Verification items for this drawing (mm, ordinates from the low corner). A direction names the side the tool comes from. Round coordinates to 2 decimals unless told otherwise and drop trailing zeros. Loops run counter-clockwise (first coordinate to the right, second up) from the corner with the lowest first, then second, coordinate; pieces in that order, holes last. Notation, with made-up numbers: M -10.5,30.25 L 45.5,30.25 A19 ccw 45.5,45.25 Z; hole C -3.75,-33.5 d11. An arc over 180 degrees is marked long. Write item = value, one per line. Start each with the question number.
(1) Go/stop test with flat-tipped pins: P1, Ø4, axis at y = 18.5, z = 5.5, coming from the +X side; P2, Ø3, axis at x = 6, z = 5, coming from the +Y side; P3, Ø3, axis at y = 4.75, z = 4, coming from the +X side; P4, Ø2.5, axis at x = 5.5, z = 5.5, coming from the +Y side. Record where each tip stops, or that it passes through.
(2) Scan lines: L1, parallel to Z at x = 1.35, y = 4.75; L2, parallel to Z at x = 7.8, y = 4.75; L3, parallel to X at y = 22.25, z = 5.5. Record each from-to range of solid material in increasing order. Write a range as from..to.
(3) Cross-section at C-C on x = 3. Record the boundary of the cut face in (y, z), plus the area to 3 significant figures.
(4) Mould release check, pull along Z, two halves, no side actions. Record for the marked faces 4, 5 and 6: pulls with the +Z half, pulls with the -Z half, needs draft (parallel to the pull), parting line crosses it, or undercut.
(5) Cross-section at A-A on y = 4.75. Record the boundary of the cut face in (x, z), plus the area to 3 significant figures.
(6) Cross-section at D-D on z = 7.25. Record the boundary of the cut face in (x, y).
(7) Cross-section at B-B on z = 4. Record the boundary of the cut face in (x, y), plus the area to 3 significant figures.
(8) Set-up check for the marked faces 1, 2 and 3: record each of +Z, -Z, +X, -X, +Y, -Y from which the full face is reachable in a straight line by a thin tool's end or side.
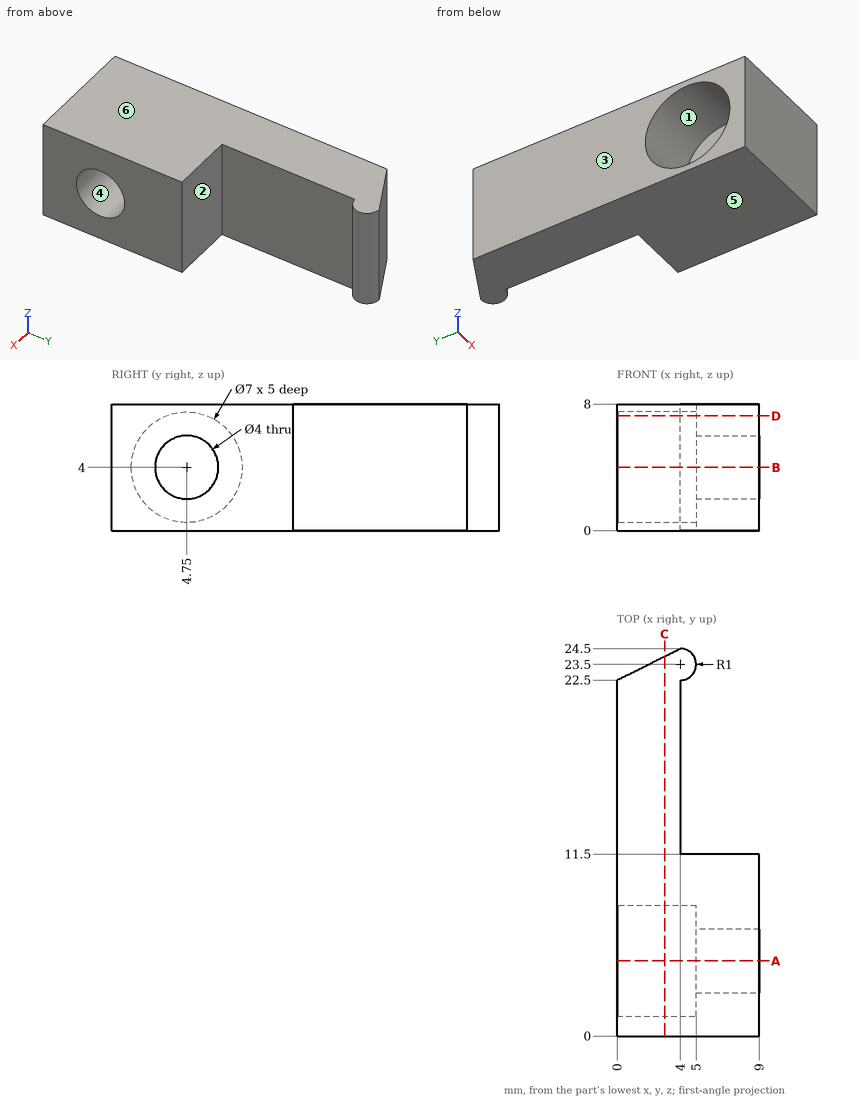
Result:
q1.P1 = 4
q1.P2 = 24.37
q1.P3 = through
q1.P4 = 24.47
q2.L1 = 0..0.5, 7.5..8
q2.L2 = 0..2, 6..8
q2.L3 = 0..4
q3.outline = M 0,0 L 24,0 L 24,8 L 0,8 Z; hole C 4.75,4 d7
q3.area = 154 mm^2
q4.face_4 = undercut
q4.face_5 = pulls with the -Z half
q4.face_6 = pulls with the +Z half
q5.outline = M 0,0 L 9,0 L 9,2 L 5,2 L 5,0.5 L 0,0.5 Z; M 0,7.5 L 5,7.5 L 5,6 L 9,6 L 9,8 L 0,8 Z
q5.area = 21.0 mm^2
q6.outline = M 0,0 L 9,0 L 9,11.5 L 4,11.5 L 4,22.5 A1 ccw 4,24.5 L 0,22.5 L 0,6.05 L 5,6.05 L 5,3.45 L 0,3.45 Z
q7.outline = M 0,0 L 9,0 L 9,2.75 L 5,2.75 L 5,1.25 L 0,1.25 Z; M 0,8.25 L 5,8.25 L 5,6.75 L 9,6.75 L 9,11.5 L 4,11.5 L 4,22.5 A1 ccw 4,24.5 L 0,22.5 Z
q7.area = 102 mm^2
q8.face_1 = -X
q8.face_2 = +Z, -Z, +X
q8.face_3 = +Z, -Z, -X, +Y, -Y
